Geometry: final body of the model. Coordinates: model frame, mm. Face numbers are marked on the shaded views. A direction names the side the tool comes from. Round coordinates to 2 decimals unless told otherwise and drop trailing zeros. Loops run counter-clockwise (first coordinate to the right, second up) from the corner with the lowest first, then second, coordinate; pieces in that order, holes last. Notation, with made-up numbers: (-21.75, 33) - (6.25, 33) arc R18 cw to (6.25, 38) - close; hole circle Ø7 at (56.5, 56). An arc over 180 degrees is marked (long way). Use CSV: the item, a comma, the result in double quotes.
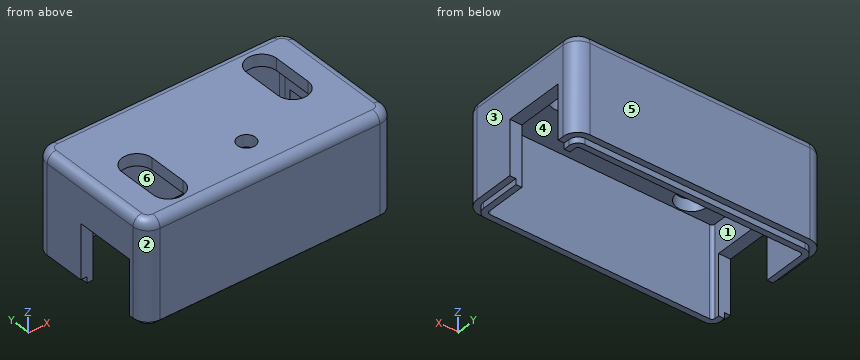
from build123d import *

# Parameters (mm, degrees)
SKETCH1_W                = 41.700000763
SKETCH1_H                = 22.799999237
BOSS_EXTRUDE1_DEPTH      = 16
BOSS_EXTRUDE1_DEPTH_BACK = 6
FILLET1_R                = 2.5
SHELL1_T                 = 2
FILLET2_R                = 1.5
SPLIT2_SURFACE_1_BACK    = 53.371
SPLIT2_SURFACE_1_DEPTH   = 106.742
SPLIT2_SURFACE_2_BACK    = 53.371
SPLIT2_SURFACE_2_DEPTH   = 106.742
SKETCH6_W                = 51.834983027
SKETCH6_H                = 10.188595942
CUT_EXTRUDE1_DEPTH       = 25
BOSS_EXTRUDE2_DEPTH      = 0.98
CUT_EXTRUDE2_DEPTH       = 11
SKETCH9_W                = 11.335588894
SKETCH9_H                = 10.028184506
CUT_EXTRUDE3_DEPTH       = 11
SKETCH10_W               = 11.009113092
SKETCH10_H               = 10.096148938
CUT_EXTRUDE4_DEPTH       = 11
SKETCH11_R               = 1.5
CUT_EXTRUDE5_DEPTH       = 11


with BuildPart() as part:
    # Sketch1 → Boss-Extrude1 (new, two sides)
    with BuildSketch(Plane.XY) as boss_extrude1_sk:
        with Locations((-17.850000382, 8.399999619)):
            Rectangle(SKETCH1_W, SKETCH1_H)
    extrude(amount=BOSS_EXTRUDE1_DEPTH)
    extrude(boss_extrude1_sk.sketch, amount=-BOSS_EXTRUDE1_DEPTH_BACK)

    # Fillet1
    fillet1_edges = [part.edges().sort_by_distance(p)[0] for p in [
        (3, -3, 5),
        (3, 19.799999237, 5),
        (-38.700000763, 19.799999237, 5),
        (-38.700000763, -3, 5),
    ]]
    fillet(fillet1_edges, radius=FILLET1_R)

    # Shell1 (no face opened: a closed hollow body)
    add(offset(amount=-SHELL1_T, mode=Mode.PRIVATE), mode=Mode.SUBTRACT)

    # Fillet2
    fillet2_edges = [part.edges().sort_by_distance(p)[0] for p in [
        (-17.850000381, -3, 16),
        (3, 8.399999619, 16),
        (-17.850000381, 19.799999237, 16),
        (-38.700000763, 8.399999619, 16),
        (-37.967767716, -2.267766953, 16),
        (-37.967767716, 19.06776619, 16),
        (2.267766953, 19.06776619, 16),
        (2.267766953, -2.267766953, 16),
    ]]
    fillet(fillet2_edges, radius=FILLET2_R)


with BuildPart() as body_2:
    # Split2: the piece behind the surface
    add(part.part)
    # Split2 surface: a surface, the sketch's curves swept straight by 106.742 mm
    with BuildLine(Plane(origin=(0, 0, 0), x_dir=(1, 0, 0), z_dir=(0, 1, 0)).offset(-SPLIT2_SURFACE_1_BACK), mode=Mode.PRIVATE) as split2_surface_1_path:
        Line((11.527694016, 0.23), (-46.74820982, 0.23))
    split2_surface_1 = Shell.extrude(split2_surface_1_path.wire(), (0 * SPLIT2_SURFACE_1_DEPTH, 1 * SPLIT2_SURFACE_1_DEPTH, 0 * SPLIT2_SURFACE_1_DEPTH))
    split(bisect_by=split2_surface_1, keep=Keep.BOTTOM)

    # Sketch6 → Cut-Extrude1 (cut)
    with BuildSketch(Plane.XZ.offset(3)):
        with Locations((-19.404183034, -5.324297971)):
            Rectangle(SKETCH6_W, SKETCH6_H)
    extrude(amount=-CUT_EXTRUDE1_DEPTH, mode=Mode.SUBTRACT)


with BuildPart() as part_1:
    add(part.part)

    # Split2: split by a surface, the side it looks to stays
    # Split2 surface: a surface, the sketch's curves swept straight by 106.742 mm
    with BuildLine(Plane(origin=(0, 0, 0), x_dir=(1, 0, 0), z_dir=(0, 1, 0)).offset(-SPLIT2_SURFACE_2_BACK), mode=Mode.PRIVATE) as split2_surface_2_path:
        Line((11.527694016, 0.23), (-46.74820982, 0.23))
    split2_surface_2 = Shell.extrude(split2_surface_2_path.wire(), (0 * SPLIT2_SURFACE_2_DEPTH, 1 * SPLIT2_SURFACE_2_DEPTH, 0 * SPLIT2_SURFACE_2_DEPTH))
    split(bisect_by=split2_surface_2, keep=Keep.TOP)

    # Sketch7 → Boss-Extrude2 (add)
    with BuildSketch(Plane(origin=(0, 0, -0.23), x_dir=(-1, 0, 0), z_dir=(0, 0, -1))):
        with BuildLine():
            Line((-0.5, -1.98), (36.200000763, -1.98))
            ThreePointArc((36.200000763, -1.98), (37.246518799, -1.546518036), (37.680000763, -0.5))
            Line((37.680000763, -0.5), (37.680000763, 17.299999237))
            ThreePointArc((37.680000763, 17.299999237), (37.246518799, 18.346517273), (36.200000763, 18.779999237))
            Line((36.200000763, 18.779999237), (-0.5, 18.779999237))
            ThreePointArc((-0.5, 18.779999237), (-1.546518036, 18.346517273), (-1.98, 17.299999237))
            Line((-1.98, 17.299999237), (-1.98, -0.5))
            ThreePointArc((-1.98, -0.5), (-1.546518036, -1.546518036), (-0.5, -1.98))
        make_face()
        with BuildLine():
            Line((-0.5, -1), (36.200000763, -1))
            ThreePointArc((36.200000763, -1), (36.553554154, -0.853553391), (36.700000763, -0.5))
            Line((36.700000763, -0.5), (36.700000763, 17.299999237))
            ThreePointArc((36.700000763, 17.299999237), (36.553554154, 17.653552628), (36.200000763, 17.799999237))
            Line((36.200000763, 17.799999237), (-0.5, 17.799999237))
            ThreePointArc((-0.5, 17.799999237), (-0.853553391, 17.653552628), (-1, 17.299999237))
            Line((-1, 17.299999237), (-1, -0.5))
            ThreePointArc((-1, -0.5), (-0.853553391, -0.853553391), (-0.5, -1))
        make_face(mode=Mode.SUBTRACT)
    extrude(amount=BOSS_EXTRUDE2_DEPTH)

    # Sketch8 → Cut-Extrude2 (cut)
    with BuildSketch(Plane.XY.offset(16)):
        with BuildLine():
            Line((-2.16, 15.093417893), (-2.16, 8.627866409))
            ThreePointArc((-2.16, 8.627866409), (-4.66, 6.127866409), (-7.16, 8.627866409))
            Line((-7.16, 8.627866409), (-7.16, 15.093417893))
            ThreePointArc((-7.16, 15.093417893), (-4.66, 17.593417893), (-2.16, 15.093417893))
        make_face()
        with BuildLine():
            Line((-33.540000763, 1.706581344), (-33.540000763, 8.172132828))
            ThreePointArc((-33.540000763, 8.172132828), (-31.040000763, 10.672132828), (-28.540000763, 8.172132828))
            Line((-28.540000763, 8.172132828), (-28.540000763, 1.706581344))
            ThreePointArc((-28.540000763, 1.706581344), (-31.040000763, -0.793418656), (-33.540000763, 1.706581344))
        make_face()
    extrude(amount=-CUT_EXTRUDE2_DEPTH, mode=Mode.SUBTRACT)

    # Sketch9 → Cut-Extrude3 (cut)
    with BuildSketch(Plane(origin=(3, 0, 0), x_dir=(0, 0, -1), z_dir=(1, 0, 0))):
        with Locations((-3.175571545, 11.266589504)):
            Rectangle(SKETCH9_W, SKETCH9_H)
    extrude(amount=-CUT_EXTRUDE3_DEPTH, mode=Mode.SUBTRACT)

    # Sketch10 → Cut-Extrude4 (cut)
    with BuildSketch(Plane.ZY.offset(38.700000763)):
        with Locations((3.338809446, 5.283196064)):
            Rectangle(SKETCH10_W, SKETCH10_H)
    extrude(amount=-CUT_EXTRUDE4_DEPTH, mode=Mode.SUBTRACT)

    # Sketch11 → Cut-Extrude5 (cut)
    with BuildSketch(Plane.XY.offset(16)):
        with Locations((-16.7, 3.3)):
            Circle(SKETCH11_R)
    extrude(amount=-CUT_EXTRUDE5_DEPTH, mode=Mode.SUBTRACT)


solid = part_1.part
Item 1: Section A-A on y = 3.3. Return the cut outline in (x, z), plus the area to 3 significant figures.
Final values:
outline,"(-38.7, 8.84) - (-36.7, 8.84) - (-36.7, 14) - (-33.54, 14) - (-33.54, 16) - (-37.2, 16) arc R1.5 ccw to (-38.7, 14.5) - close; (-28.54, 14) - (-18.2, 14) - (-18.2, 16) - (-28.54, 16) - close; (-15.2, 14) - (1, 14) - (1, -1.21) - (1.98, -1.21) - (1.98, -0.23) - (3, -0.23) - (3, 14.5) arc R1.5 ccw to (1.5, 16) - (-15.2, 16) - close"
area,"106 mm²"
Item 2: Mould query, pull axis X, two halves, no side actions, for the marked faces 3, 4, 5 and 6. Classes: released by +X, released by -X, zero draft, split by the parting line, or undercut.
Final values:
face 3,"released by +X"
face 4,"undercut"
face 5,"zero draft"
face 6,"undercut"
Item 3: Section D-D on y = 13.5. Return the cut outline in (x, z).
Final values:
outline,"(-38.7, -0.23) - (-37.68, -0.23) - (-37.68, -1.21) - (-36.7, -1.21) - (-36.7, 14) - (-7.16, 14) - (-7.16, 16) - (-37.2, 16) arc R1.5 ccw to (-38.7, 14.5) - close; (-2.16, 14) - (1, 14) - (1, 8.84) - (3, 8.84) - (3, 14.5) arc R1.5 ccw to (1.5, 16) - (-2.16, 16) - close"
Item 4: Pin query (flat end, axial travel): P1, Ø1, axis at y = 11.5, z = 15.5, coming from the -X side; P2, Ø1.6, axis at x = -37.5, z = 2.5, coming from the +Y side; P3, Ø6, axis at x = -15, y = 10, coming from the -Z side. Return the tip coordinate at first contact, or that it passes through.
Final values:
P1,"stops at x = -38.61"
P2,"stops at y = 19.75"
P3,"stops at z = 14"
Item 5: Section C-C on z = 11. Return the cut outline in (x, y).
Final values:
outline,"(-38.7, -0.5) arc R2.5 ccw to (-36.2, -3) - (0.5, -3) arc R2.5 ccw to (3, -0.5) - (3, 17.3) arc R2.5 ccw to (0.5, 19.8) - (-36.2, 19.8) arc R2.5 ccw to (-38.7, 17.3) - close; hole (-36.7, -0.5) arc R0.5 ccw to (-36.2, -1) - (0.5, -1) arc R0.5 ccw to (1, -0.5) - (1, 17.3) arc R0.5 ccw to (0.5, 17.8) - (-36.2, 17.8) arc R0.5 ccw to (-36.7, 17.3) - close"
Item 6: Section B-B on x = -4.66. Return the cut outline in (y, z).
Final values:
outline,"(-3, -0.23) - (-1.98, -0.23) - (-1.98, -1.21) - (-1, -1.21) - (-1, 14) - (6.13, 14) - (6.13, 16) - (-1.5, 16) arc R1.5 ccw to (-3, 14.5) - close; (17.59, 14) - (17.8, 14) - (17.8, -1.21) - (18.78, -1.21) - (18.78, -0.23) - (19.8, -0.23) - (19.8, 14.5) arc R1.5 ccw to (18.3, 16) - (17.59, 16) - close"
Item 7: Reachability of the marked faces 1 and 2 from +Z, -Z, +X, -X, +Y, -Y: full face, straight path, thin tool, end or side. Return the list, or none.
Final values:
face 1,"-Z"
face 2,"+Z, -Z, -X, -Y"
Item 8: Material intervals for line 1 (Y direction, x = -18, z = 12.5); line 2 (X direction, y = 12.25, z = 11.25); line 3 (X direction, y = 7.75, z = 14.5), sorted ascending.
Final values:
line 1,"y = -3 to -1, 17.8 to 19.8"
line 2,"x = -38.7 to -36.7, 1 to 3"
line 3,"x = -38.7 to -33.54, -28.54 to -7, -2.32 to 3"
